The model under review builds one solid part; all positions refer to its coordinate system, in mm. A direction names the side the tool comes from. Round coordinates to 2 decimals unless told otherwise and drop trailing zeros. Write each loop counter-clockwise with the first axis right and the second up, starting at its lowest first coordinate (ties: lowest second). Pieces come first, ordered by that corner, then holes. Notation, with made-up numbers: (-15, 54) -> (21, 54) arc R29 ccw to (21, 86) -> close; hole circle Ø9 at (-29, 24). An arc over 180 degrees is marked (long way). Answer as a JSON object with one key per item and string values. Group by question number.
1) Machinability: for faces 1 (the flat face through (35, -13, 12.7)), 2 (the cylindrical face through (56.797, -12.421, 6.439)), 3 (the flat face through (6, -19.252, 37)), which of the approach directions +Z, -Z, +X, -X, +Y, -Y give a long, thin tool a straight path to every point of the face, cutting with its end or side? Answer none if there is none.
2) Mouldability with a two-part tool opening along Y and no side actions: class faces 4 (the flat face through (21.7, -12.5, 0)), 5 (the cylindrical face through (6.44, -2.04, 42.65)), 6 (the cylindrical face through (6.439, -13.041, 22.227)) as pulls with the +Y half, pulls with the -Y half, needs draft (parallel to the pull), parting line crosses it, or undercut.
3) We need section C-C, the plane z = 37. Write out the cut boundary in (x, y).
4) We need section A-A, the plane x = 27. Write out the cut boundary in (y, z), then the cut area to 3 significant figures.
5) Insertion check: pin 1 Ø4 at (y, z) = (-8, 31.5) entering from +X; pin 2 Ø12.5 at (x, y) = (31.5, -10) entering from +Z; pin 3 Ø2 at (y, z) = (-7, 7.5) entering from +X. Each pin has a flat end and moves straight along its axis. Give the tip position at first contact, or say it passes through.
6) To check wall thickness, follow probe 1 along X at (y, z) = (-9, 11); probe 2 along X at (y, z) = (-4.5, 17.5). State the ranges of each line that lie inside material, in increasing order. Write a range as [from, to].
7) We need section B-B, the plane y = -7.5. Write out the cut boundary in (x, z).
from build123d import *

# Parameters (mm, degrees)
F1_DEPTH = 25.4
F3_DEPTH = 12.7
F4_R     = 6.35
F5_DEPTH = 12.7


with BuildPart() as f1:
    # F0 (on Front) → F1 (new body)
    with BuildSketch(Plane.XZ):
        Polygon((0, 44.45), (0, 0), (57.15, 0), (57.15, 12.7), (12.7, 12.7), (12.7, 44.45), align=None)
    extrude(amount=F1_DEPTH)

    # F2 (on face) → F3 (cut)
    with BuildSketch(Plane.YZ.offset(12.7)):
        with BuildLine():
            ThreePointArc((-19.2516389379, 28.575), (-12.9016389379, 22.225), (-6.5516389379, 28.575))
            ThreePointArc((-6.5516389379, 28.575), (-12.9016389379, 34.925), (-19.2516389379, 28.575))
        make_face()
        with BuildLine():
            ThreePointArc((-19.2516389379, 28.575), (-12.9016389379, 34.925), (-6.5516389379, 28.575))
            Line((-6.5516389379, 28.575), (-6.5516389379, 44.45))
            Line((-6.5516389379, 44.45), (-19.2516389379, 44.45))
            Line((-19.2516389379, 44.45), (-19.2516389379, 28.575))
        make_face()
        with BuildLine():
            Line((0, 44.45), (-6.5516389379, 44.45))
            ThreePointArc((-6.5516389379, 44.45), (-1.9896636866, 42.6019965832), (0, 38.1))
            Line((0, 38.1), (0, 44.45))
        make_face()
        with BuildLine():
            ThreePointArc((-25.4, 39.6875), (-23.1402039046, 43.1201157855), (-19.2516389379, 44.45))
            Line((-19.2516389379, 44.45), (-25.4, 44.45))
            Line((-25.4, 44.45), (-25.4, 39.6875))
        make_face()
    extrude(amount=-F3_DEPTH, mode=Mode.SUBTRACT)

    # F4 (on face) → F5 (cut)
    with BuildSketch(Plane.XY.offset(12.7)):
        with Locations((28.2040209995, -11.4295053813)):
            Circle(F4_R)
        with Locations((44.1000172256, -11.2356515601)):
            Circle(F4_R)
        with BuildLine():
            ThreePointArc((44.1000172256, 0), (56.8000172256, -12.7), (44.1000172256, -25.4))
            Line((44.1000172256, -25.4), (57.15, -25.4))
            Line((57.15, -25.4), (57.15, 0))
            Line((57.15, 0), (44.1000172256, 0))
        make_face()
    extrude(amount=-F5_DEPTH, mode=Mode.SUBTRACT)


solid = f1.part
Here are the results:
{
 "1": {"face 1": "+Z, +X, +Y, -Y", "face 2": "+Z, -Z, +X", "face 3": "+Z, +X, -X"},
 "2": {"face 4": "needs draft", "face 5": "pulls with the +Y half", "face 6": "undercut"},
 "3": {"outline": "(0, -25.4) -> (12.7, -25.4) -> (12.7, -19.25) -> (0, -19.25) -> close; (0, -6.55) -> (12.7, -6.55) -> (12.7, 0) -> (0, 0) -> close"},
 "4": {"outline": "(-25.4, 0) -> (-17.66, 0) -> (-17.66, 12.7) -> (-25.4, 12.7) -> close; (-5.19, 0) -> (0, 0) -> (0, 12.7) -> (-5.19, 12.7) -> close", "area": "164 mm^2"},
 "5": {"pin 1": "stops at x = 12.7", "pin 2": "stops at z = 12.7", "pin 3": "stops at x = 55.9"},
 "6": {"probe 1": "x = [0, 22.34], [34.07, 38.16], [50.04, 56.25]", "probe 2": "x = [0, 12.7]"},
 "7": {"outline": "(0, 0) -> (23.22, 0) -> (23.22, 12.7) -> (12.7, 12.7) -> (12.7, 25.24) -> (0, 25.24) -> close; (33.19, 0) -> (38.97, 0) -> (38.97, 12.7) -> (33.19, 12.7) -> close; (49.23, 0) -> (55.69, 0) -> (55.69, 12.7) -> (49.23, 12.7) -> close"}
}
